from build123d import *

# Parameters (mm, degrees)
F5_D           = 4.4958
F5_START       = 1.27
F5_CSINK_D     = 9.1186
F5_CSINK_ANGLE = 82
F9_D           = 5.1054
F9_CBORE_D     = 7.9375
F9_CBORE_DEPTH = 4.826


# Not quite as in the source:
# - a feature names something its author has since deleted; it is built from what else it names


with BuildPart() as f2:
    # F2: sweep along a path in F0
    with BuildLine(Plane.XZ) as f2_path:
        Line((384.6068, 55.8292), (0, 55.8292))
    # F1 (on Right) → F2 (sweep)
    with BuildSketch(Plane.YZ):
        with BuildLine():
            Line((15.875, 54.5592), (0, 54.5592))
            Line((0, 54.5592), (-15.875, 54.5592))
            Line((-15.875, 54.5592), (-15.875, 55.8292))
            Line((-15.875, 55.8292), (-22.225, 55.8292))
            Line((-22.225, 55.8292), (-15.6786488693, 46.3042))
            Line((-15.6786488693, 46.3042), (-15.6786488693, 36.7792))
            Line((-15.6786488693, 36.7792), (-7.2411052202, 36.7792))
            ThreePointArc((-7.2411052202, 36.7792), (0, 47.9679), (7.2411052202, 36.7792))
            Line((7.2411052202, 36.7792), (15.6786488693, 36.7792))
            Line((15.6786488693, 36.7792), (15.6786488693, 46.3042))
            Line((15.6786488693, 46.3042), (22.225, 55.8292))
            Line((22.225, 55.8292), (15.875, 55.8292))
            Line((15.875, 55.8292), (15.875, 54.5592))
        make_face()
    sweep(path=f2_path.line)

    # F5 (through all)
    # its depths count from where the whole tool has entered the part; down to there all is cleared
    with Locations(Plane.XY.offset(55.8292).offset(-F5_START)):
        with Locations((359.2068, 0)):
            CounterSinkHole(F5_D / 2, F5_CSINK_D / 2, counter_sink_angle=F5_CSINK_ANGLE)

    # F9 (through all)
    with Locations(Plane.XY.offset(54.5592)):
        with Locations((60.325, 11.4598770448), (60.325, -11.4598770448), (19.05, -11.4598770448), (19.05, 11.4598770448)):
            CounterBoreHole(F9_D / 2, F9_CBORE_D / 2, F9_CBORE_DEPTH)


solid = f2.part
Model file for the job. Use its own axes, mm. A direction names the side the tool comes from. Give positions to 0.01 mm unless a question says otherwise; leave off trailing zeros. Order: outer loops, then holes, each group sorted by start corner. A loop starts at its lowest first (then second) coordinate and runs counter-clockwise, first axis right, second up. Notation, with made-up numbers: (-12.75, 42) - (13.25, 42) arc R28 cw to (13.25, 79) - close; hole circle Ø2 at (28, 76.5). An arc over 180 degrees is marked (long way). Return JSON: item names as keys, results as strings.
1) Flat gauge pins, fed straight in: P1, Ø1, axis at x = 203.5, z = 55, coming from the +Y side; P2, Ø3, axis at x = 293.5, z = 42.5, coming from the +Y side; P3, Ø3, axis at x = 105, z = 40.5, coming from the -Y side; P4, Ø3.5, axis at x = 359.21, y = 0, coming from the +Z side. Where does each tip first touch, or does it go through?
Geometry says:
{"P1": "y = 22", "P2": "y = 15.68", "P3": "y = -15.68", "P4": "through"}
2) Pull direction X, two halves, no side cores. Call faces 5 (the flat face through (0, -0.3, 48.3)), 6 (the conical face through (356.956, 0.709, 52.029)), 7 (the flat face through (189.611, 18.906, 51)): pulls with the +X half, pulls with the -X half, needs draft (parallel to the pull), parting line crosses it, or undercut.
Geometry says:
{"face 5": "pulls with the -X half", "face 6": "undercut", "face 7": "needs draft"}
3) Cut at B-B, the plane x = 283. Give the cut face in (y, z) (1 decimal).
Geometry says:
{"outline": "(-22.2, 55.8) - (-15.7, 46.3) - (-15.7, 36.8) - (-7.2, 36.8) arc R7.9 cw (long way) to (7.2, 36.8) - (15.7, 36.8) - (15.7, 46.3) - (22.2, 55.8) - (15.9, 55.8) - (15.9, 54.6) - (-15.9, 54.6) - (-15.9, 55.8) - close"}
4) Probe line 1 (X direction, y = -11.5, z = 41.5); line 2 (X direction, y = 12, z = 45.5); line 3 (Y direction, x = 58.5, z = 42.25). List the from-to ranges inside material, lowest first. Write a range as from..to.
Geometry says:
{"line 1": "0..16.5, 21.6..57.77, 62.88..384.61", "line 2": "0..16.56, 21.54..57.83, 62.82..384.61", "line 3": "-15.68..-13.24, -9.68..-7.62, 7.62..9.68, 13.24..15.68"}
5) Cut at A-A, the plane z = 43.25. Give the cut face in (x, y) (3 decimals), plus the area to 3 significant figures.
Geometry says:
{"outline": "(0, -15.679) - (384.607, -15.679) - (384.607, -7.255) - (0, -7.255) - close; (0, 7.255) - (384.607, 7.255) - (384.607, 15.679) - (0, 15.679) - close; hole circle Ø5.105 at (19.05, -11.46); hole circle Ø5.105 at (19.05, 11.46); hole circle Ø5.105 at (60.325, -11.46); hole circle Ø5.105 at (60.325, 11.46)", "area": "6,400 mm²"}
6) 3-axis set-ups, long thin cutter, end or side, ignore diameter. For faces 1 (the flat face through (190, 15.679, 41)), 2 (the flat face through (190, 0, 54.559)), 3 (the flat face through (190, -12, 36.779)), 4 (the cylindrical face through (15.085, -11.285, 52.18)): which of +Z, -Z, +X, -X, +Y, -Y reach the whole face in a straight line?
Geometry says:
{"face 1": "-Z, +X, -X, +Y", "face 2": "+Z, +X, -X", "face 3": "-Z, +X, -X, +Y, -Y", "face 4": "+Z"}
